Check sheet for the modelled part. Datum: model origin and axes. Units: mm. Face numbers are marked on the shaded views. A direction names the side the tool comes from. Give positions to 0.01 mm unless a question says otherwise; leave off trailing zeros. Write each loop counter-clockwise with the first axis right and the second up, starting at its lowest first coordinate (ties: lowest second). Pieces come first, ordered by that corner, then holes. Notation, with made-up numbers: M -31.5,-40 L -16.5,-40 A24 cw -16.5,-1 Z; hole C 75,-8 d4. An arc over 180 degrees is marked long. One line per item, written item: value. Start each with the question number.
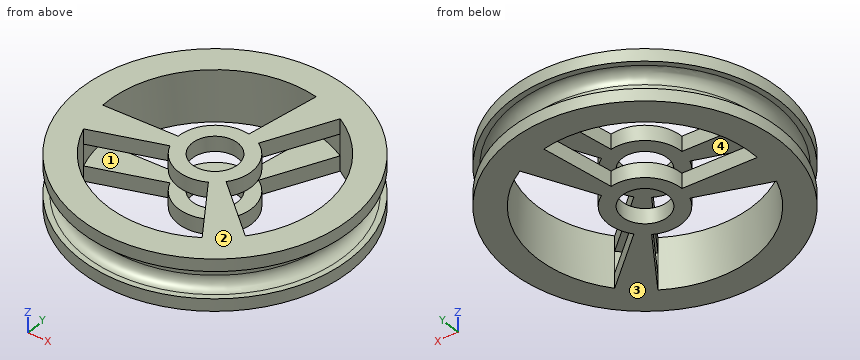
from build123d import *
from build123d import SkipClean  # not in build123d's __all__

# Parameters (mm, degrees)
F0_R     = 15.875
F1_DEPTH = 3.048
F2_R     = 17.9958283003
F2_R_2   = 13.97
F3_DEPTH = 1.5875
F4_R     = 2.667
F5_DEPTH = 6.097
F6_R     = 1.27
F7_R     = 12.7
F8_DEPTH = 1.27


with BuildPart() as f1:
    # F0 (on Top) → F1 (new body, symmetric)
    with BuildSketch(Plane.XY):
        Circle(F0_R)
    extrude(amount=F1_DEPTH, both=True)

    # F2 (on Top) → F3 (cut, symmetric)
    with BuildSketch(Plane.XY):
        Circle(F2_R)
        Circle(F2_R_2, mode=Mode.SUBTRACT)
    extrude(amount=F3_DEPTH, both=True, mode=Mode.SUBTRACT)

    # F4 (on face) → F5 (cut, through all)
    with BuildSketch(Plane.XY.offset(3.048)):
        with BuildLine():
            Line((0.6120390991, 4.2744043025), (2.0170417977, 12.5388014733))
            ThreePointArc((2.0170417977, 12.5388014733), (-8.4665969818, 9.4660834323), (-12.6852858441, -0.6111653244))
            Line((-12.6852858441, -0.6111653244), (-4.318, 0))
            ThreePointArc((-4.318, 0), (-2.8286338726, 3.2625073816), (0.6120390991, 4.2744043025))
        make_face()
        Circle(F4_R)
        with BuildLine():
            ThreePointArc((2.159, -3.7394976935), (-1.4110973362, -4.0809224824), (-4.0077622616, -1.6071607433))
            Line((-4.0077622616, -1.6071607433), (-11.8674415077, -4.5225912993))
            ThreePointArc((-11.8674415077, -4.5225912993), (-3.9645702358, -12.065329786), (6.8719276189, -10.6801971331))
            Line((6.8719276189, -10.6801971331), (2.159, -3.7394976935))
        make_face()
        with BuildLine():
            ThreePointArc((2.159, 3.7394976935), (4.2397312088, 0.8184151008), (3.3957231624, -2.6672435592))
            Line((3.3957231624, -2.6672435592), (9.85039971, -8.016210174))
            ThreePointArc((9.85039971, -8.016210174), (12.4311672176, 2.5992463537), (5.8133582252, 11.2913624574))
            Line((5.8133582252, 11.2913624574), (2.159, 3.7394976935))
        make_face()
    extrude(amount=-F5_DEPTH, mode=Mode.SUBTRACT)

    # F6
    f6_edges = [f1.edges().sort_by_distance(p)[0] for p in [
        (-13.97, 0, -1.5875),
        (-13.97, 0, 1.5875),
    ]]
    fillet(f6_edges, radius=F6_R)

    # F7 (on Top) → F8 (cut, symmetric)
    with BuildSketch(Plane.XY):
        Circle(F7_R)
    with SkipClean():  # cleaning this boolean's faces spoils the solid; the shape is the same uncleaned
        extrude(amount=F8_DEPTH, both=True, mode=Mode.SUBTRACT)


solid = f1.part
1) Gauge pin test, flat ends, axial feed: pin 1 (3 mm diameter, centred on x = 0, y = 0, fed in from -Z); pin 2 (2 mm diameter, centred on x = 4, z = 2.5, fed in from -Y). Record the tip position at first contact, or that the pin passes through.
2) Tool access check on the marked faces 3 and 4. Record the directions out of +Z, -Z, +X, -X, +Y, -Y that give a thin tool (end or side, any length) a straight path to the whole face; none if there is none.
3) Material ranges on L1, parallel to Y at x = 0, z = 1.75 (3 decimals); L2, parallel to Y at x = 3, z = 2.25; L3, parallel to Y at x = -11, z = 2.5, recorded low to high. Write a range as from..to.
4) Cross-section at A-A (z = -2.25). State how many separate pieces and enclosed holes the cut face has, plus the area to 3 significant figures.
5) Draft check along X on the marked faces 1 and 2. Enter one of: released by +X, released by -X, zero draft, split by the parting line, or undercut.
6) Cross-section at B-B (z = 0.75). Record the boundary of the cut face in (x, y), plus the area to 3 significant figures.
Data:
1. pin 1: passes through
1. pin 2: stops at y = -15.59
2. face 3: -Z, +X, -X, +Y, -Y
2. face 4: none
3. L1: y = -15.875..-12.7, -4.318..-2.667, 2.667..4.318, 12.7..15.875
3. L2: y = -15.59..-12.34, -4.98..3.11, 5.48..15.59
3. L3: y = -11.45..-6.35, -4.2..-0.49, 6.35..11.45
4. separate pieces: 1
4. enclosed holes: 4
4. area: 392 mm2
5. face 1: undercut
5. face 2: zero draft
6. outline: C 0,0 d28.09; hole C 0,0 d25.4
6. area: 113 mm2
